from build123d import *

# Parameters (mm, degrees)
ESQUISSE1_R             = 2.5
BOSS_EXTRU_1_DEPTH      = 20
ESQUISSE2_R             = 1.5
BOSS_EXTRU_2_DEPTH      = 6
ESQUISSE6_R             = 1.7
ENL_V_MAT_EXTRU_1_DEPTH = 10


with BuildPart() as part:
    # Esquisse1 → Boss.-Extru.1 (new body)
    with BuildSketch(Plane(origin=(0, 0, 0), x_dir=(1, 0, 0), z_dir=(0, 1, 0))):
        Circle(ESQUISSE1_R)
    extrude(amount=BOSS_EXTRU_1_DEPTH)

    # Esquisse2 → Boss.-Extru.2 (add)
    with BuildSketch(Plane.XZ):
        Circle(ESQUISSE2_R)
    extrude(amount=BOSS_EXTRU_2_DEPTH)

    # Esquisse6 → Enlèv. mat.-Extru.1 (cut)
    with BuildSketch(Plane(origin=(0, 20, 0), x_dir=(1, 0, 0), z_dir=(0, 1, 0))):
        Circle(ESQUISSE6_R)
    extrude(amount=-ENL_V_MAT_EXTRU_1_DEPTH, mode=Mode.SUBTRACT)


solid = part.part
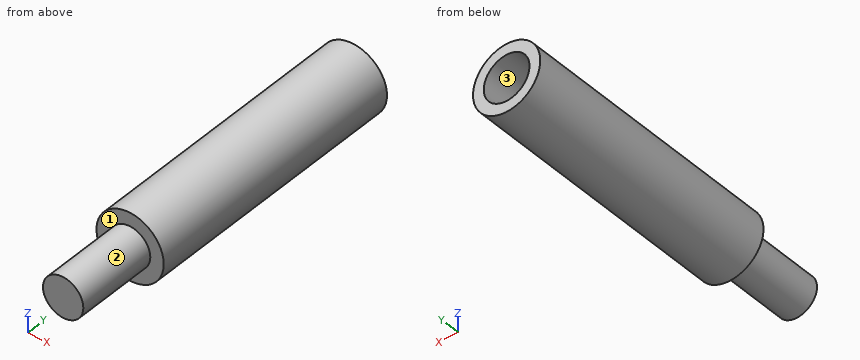
Source: CAD feature listing. Evaluate the final solid. Frame: model axes, mm. Face numbers are marked on the shaded views. Give positions to 0.01 mm unless a question says otherwise; leave off trailing zeros. Write each loop counter-clockwise with the first axis right and the second up, starting at its lowest first coordinate (ties: lowest second). Pieces come first, ordered by that corner, then holes. Notation, with made-up numbers: (56, 31) -> (82, 31) arc R18 cw to (82, 60) -> close; hole circle Ø7 at (62.25, 4). An arc over 180 degrees is marked (long way). Write item = value, one per line.
Q1. Mould query, pull axis X, two halves, no side actions, for the marked faces 1, 2 and 3. Classes: +X half, -X half, draft (parallel to the pull), parting line (faces both ways), or undercut.
Here are the results:
face_1 = draft
face_2 = parting line
face_3 = undercut
Q2. Cut plane C-C on y = 5.75. Return loops of the section in (x, z).
Here are the results:
outline = circle Ø5 at (0, 0)
Q3. Cut plane A-A on x = 0. Return loops of the section in (y, z), then the cut area to 3 significant figures.
Here are the results:
outline = (-6, -1.5) -> (0, -1.5) -> (0, -2.5) -> (20, -2.5) -> (20, -1.7) -> (10, -1.7) -> (10, 1.7) -> (20, 1.7) -> (20, 2.5) -> (0, 2.5) -> (0, 1.5) -> (-6, 1.5) -> close
area = 84.0 mm²
Q4. Cut plane B-B on z = 0. Return loops of the section in (x, y), then the cut area to 3 significant figures.
Here are the results:
outline = (-2.5, 0) -> (-1.5, 0) -> (-1.5, -6) -> (1.5, -6) -> (1.5, 0) -> (2.5, 0) -> (2.5, 20) -> (1.7, 20) -> (1.7, 10) -> (-1.7, 10) -> (-1.7, 20) -> (-2.5, 20) -> close
area = 84.0 mm²
Q5. Cut plane D-D on y = -0.5. Return loops of the section in (x, z).
Here are the results:
outline = circle Ø3 at (0, 0)
Q6. Line query: line 1 (Z direction, x = 0, y = 18.25); line 2 (Y direction, x = 2.1, z = -1). Output: solid intervals per line, ascending. Write a range as from..to.
Here are the results:
line_1 = -2.5..-1.7, 1.7..2.5
line_2 = 0..20
Q7. First-contact query: pin 1 (1 mm diameter, centred on x = -1, y = 12, fed in from +Z); pin 2 (1.5 mm diameter, centred on y = 11, z = 1, fed in from +X). Flat tips, straight axial feed; report the tip coordinate or a pass-through.
Here are the results:
pin_1 = 2.45
pin_2 = 2.49
